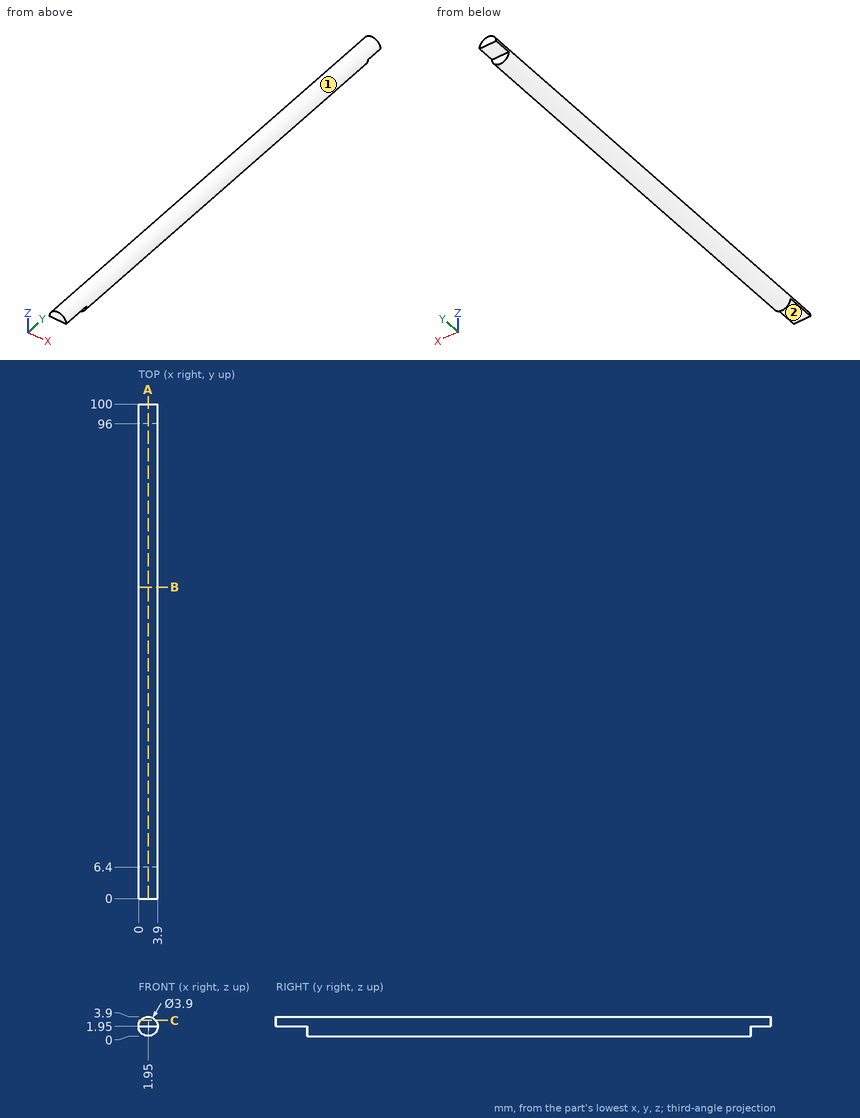
Design review of the part shown in the three views and the two pictorial views. Dimensions are in mm from the part's minimum x, y and z. A direction names the side the tool comes from. Round coordinates to 2 decimals unless told otherwise and drop trailing zeros. Write each loop counter-clockwise with the first axis right and the second up, starting at its lowest first coordinate (ties: lowest second). Pieces come first, ordered by that corner, then holes.
Item 1: We need section C-C on z = 3.15. Write out the cut boundary in (x, y), and give its area (3 significant figures).
Item 2: For the marked faces 1 and 2, list the 3-axis set-ups (+Z, -Z, +X, -X, +Y, -Y) from which the entire face can be reached by the end or side of a thin tool; tool diameter is ignored.
Item 3: For probe 1 along Y at (x, z) = (2, 0.8); probe 2 along X at (y, z) = (36.5, 1.75); probe 3 along Z at (x, y) = (2, 5), list the stretches that pass through material, from the lowest coordinate up.
Item 4: We need section A-A on x = 1.95. Write out the cut boundary in (y, z), and give its area (3 significant figures).
Item 5: We need section B-B on y = 63. Write out the cut boundary in (x, z), and give its area (3 significant figures).
Item 6: Clearance check with flat-ended pins moving along their axes: pin 1 Ø1.6 at (x, z) = (2, 1) entering from -Y; pin 2 Ø1.5 at (x, z) = (3.5, 0.5) entering from +Y. State where each tip first meets the part, or that it passes through.
Returned:
1. outline: (0.41, 0) - (3.49, 0) - (3.49, 100) - (0.41, 100) - close
1. area: 307 mm2
2. face 1: +Y, -Y
2. face 2: -Z, +X, -X, -Y
3. probe 1: y = 6.4 to 96
3. probe 2: x = 0.01 to 3.89
3. probe 3: z = 1.95 to 3.9
4. outline: (0, 1.95) - (6.4, 1.95) - (6.4, 0) - (96, 0) - (96, 1.95) - (100, 1.95) - (100, 3.9) - (0, 3.9) - close
4. area: 370 mm2
5. outline: circle Ø3.9 at (1.95, 1.95)
5. area: 11.9 mm2
6. pin 1: stops at y = 6.4
6. pin 2: stops at y = 96
